Drawing for the job (mm, zero at the part's lowest x, y, z). Round coordinates to 2 decimals unless told otherwise and drop trailing zeros. Order: outer loops, then holes, each group sorted by start corner. A loop starts at its lowest first (then second) coordinate and runs counter-clockwise, first axis right, second up. Notation, with made-up numbers: (-16.5, 26.25) -> (12.5, 26.25) arc R19 cw to (12.5, 53.25) -> close; hole circle Ø9 at (52.25, 5). An arc over 180 degrees is marked (long way). Use CSV: the item, a comma, the result in double quotes.
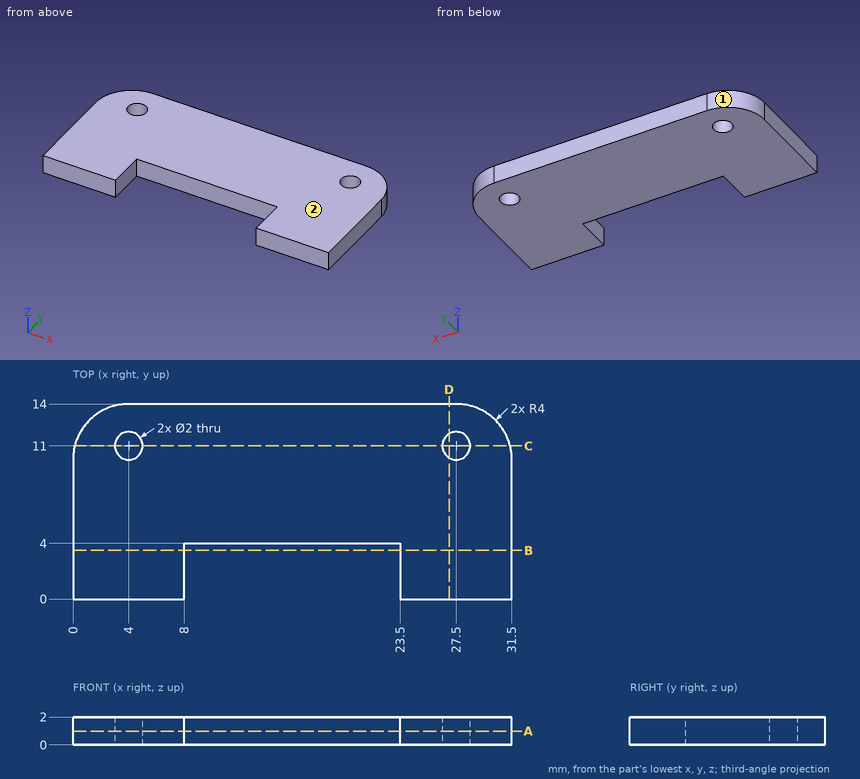
Q1. Mould opens along Y. For the marked faces 1 and 2 say: +Y half, -Y half, draft (parallel to the pull), parting line (faces both ways), or undercut.
From the geometry:
face 1,"+Y half"
face 2,"draft"
Q2. Cut at B-B (y = 3.5). Give the cut face in (x, z).
From the geometry:
outline,"(0, 0) -> (8, 0) -> (8, 2) -> (0, 2) -> close; (23.5, 0) -> (31.5, 0) -> (31.5, 2) -> (23.5, 2) -> close"
Q3. Cut at D-D (x = 27). Give the cut face in (y, z), plus the area to 3 significant figures.
From the geometry:
outline,"(0, 0) -> (10.13, 0) -> (10.13, 2) -> (0, 2) -> close; (11.87, 0) -> (14, 0) -> (14, 2) -> (11.87, 2) -> close"
area,"24.5 mm²"
Q4. Cut at C-C (y = 11). Give the cut face in (x, z).
From the geometry:
outline,"(0.13, 0) -> (3, 0) -> (3, 2) -> (0.13, 2) -> close; (5, 0) -> (26.5, 0) -> (26.5, 2) -> (5, 2) -> close; (28.5, 0) -> (31.37, 0) -> (31.37, 2) -> (28.5, 2) -> close"
Q5. Pin check, flat tip, straight feed: pin 1 (1 mm diameter, centred on x = 18.5, z = 0.5, fed in from -Y). Stop position of the tip, or through.
From the geometry:
pin 1,"stops at y = 4"
Q6. Cut at A-A (z = 1). Give the cut face in (x, y), plus the area to 3 significant figures.
From the geometry:
outline,"(0, 0) -> (8, 0) -> (8, 4) -> (23.5, 4) -> (23.5, 0) -> (31.5, 0) -> (31.5, 10) arc R4 ccw to (27.5, 14) -> (4, 14) arc R4 ccw to (0, 10) -> close; hole circle Ø2 at (4, 11); hole circle Ø2 at (27.5, 11)"
area,"366 mm²"
Q7. Probe line 1 along X through (y, z) = (2.25, 0.45); line 2 along Y through (x, z) = (4, 1.45); line 3 along Y through (x, z) = (12.5, 0.5). List the from-to ranges inside material, lowest first.
From the geometry:
line 1,"x = 0 to 8, 23.5 to 31.5"
line 2,"y = 0 to 10, 12 to 14"
line 3,"y = 4 to 14"
